from build123d import *

# Parameters (mm, degrees)
PAD_DEPTH       = 32
POCKET_DEPTH    = 27
SKETCH021_R     = 62.5
POCKET014_DEPTH = 29


with BuildPart() as part:
    # Sketch → Pad (new body)
    with BuildSketch(Plane.XY):
        with BuildLine():
            ThreePointArc((-51.234754, 40), (0, -65), (51.234754, 40))
            ThreePointArc((51.234754, 120), (37.469508, 80), (51.234754, 40))
            ThreePointArc((51.234754, 120), (0, 225), (-51.234754, 120))
            ThreePointArc((-51.234754, 40), (-37.469508, 80), (-51.234754, 120))
        make_face()
    extrude(amount=PAD_DEPTH)

    # Sketch001 (on Face6 of Pad) → Pocket (cut)
    with BuildSketch(Plane.XY.offset(32)):
        with BuildLine():
            ThreePointArc((-47.293673, 36.923008), (4.4e-05, -60), (47.293619, 36.923077))
            ThreePointArc((47.293619, 123.076923), (32.469508, 80), (47.293619, 36.923077))
            ThreePointArc((47.293619, 123.076923), (0, 220), (-47.293619, 123.076923))
            ThreePointArc((-47.293673, 36.923008), (-32.469508, 79.999956), (-47.293619, 123.076923))
        make_face()
    extrude(amount=-POCKET_DEPTH, mode=Mode.SUBTRACT)

    # Sketch021 (on Face5 of Pocket) → Pocket014 (cut)
    with BuildSketch(Plane.XY.offset(32)):
        Circle(SKETCH021_R)
    extrude(amount=-POCKET014_DEPTH, mode=Mode.SUBTRACT)


solid = part.part
Read the model definition and answer for the solid it produces. Units are mm, in the model's axes. A direction names the side the tool comes from. Round coordinates to 2 decimals unless told otherwise and drop trailing zeros. Write each loop counter-clockwise with the first axis right and the second up, starting at its lowest first coordinate (ties: lowest second). Pieces come first, ordered by that corner, then holes.
1. Which of the six approach directions +Z, -Z, +X, -X, +Y, -Y give full straight-line access (tool end or side, diameter ignored) to faces 3 (the face through (32.82, 86.98, 18.69)), 4 (the face through (38, 102, 32))?
2. Determine the mould class of faces 1 (the face through (-1, 1, 3)), 2 (the face through (-1, 82, 0)) for opening direction Y: pulls with the +Y half, pulls with the -Y half, needs draft (parallel to the pull), parting line crosses it, or undercut.
3. Given pin 1 Ø10 at (y, z) = (56, 25) entering from -X; pin 2 Ø5 at (x, y) = (-12.5, 70) entering from +Z; pin 3 Ø8 at (x, z) = (47, 16.5) entering from +Y, each flat-ended and moving along its own axis, determine where each tip first touches the part or whether it passes through.
4. Straight lines are drawn through the part: L1, parallel to Y at x = 0, z = 11; L2, parallel to Y at x = 45, z = 20.5; L3, parallel to X at y = 160, z = 26.75. For each, find the intervals that lie inside material, in ascending order.
5. The part is cut by section B-B, the plane y = 0. Determine the outline of the cut face in (x, z), then the cut area to 3 significant figures.
6. The part is cut by section C-C, the plane z = 28.5. Determine the outline of the cut face in (x, y).
7. The part is cut by section A-A, the plane x = 0. Determine the outline of the cut face in (y, z).
8. The part is cut by section D-D, the plane y = 160. Determine the outline of the cut face in (x, z).
Values:
1. face 3: +Z
1. face 4: +Z, +X, -X, +Y, -Y
2. face 1: undercut
2. face 2: needs draft
3. pin 1: stops at x = -44.3
3. pin 2: stops at z = 5
3. pin 3: stops at y = 208.74
4. L1: y = -65 to -62.5, 220 to 225
4. L2: y = -46.9 to -43.37, 43.37 to 49.63, 110.37 to 119.97, 199.69 to 206.9
4. L3: x = -65 to -60, 60 to 65
5. outline: (-65, 0) - (65, 0) - (65, 32) - (62.5, 32) - (62.5, 3) - (-62.5, 3) - (-62.5, 32) - (-65, 32) - close
5. area: 535 mm2
6. outline: (-51.23, 40) arc R65 ccw (long way) to (51.23, 40) arc R65 cw to (51.23, 120) arc R65 ccw (long way) to (-51.23, 120) arc R65 cw to start; hole (-47.29, 123.08) arc R70 cw to (-40.35, 47.73) arc R62.5 ccw (long way) to (40.35, 47.73) arc R70 cw to (47.29, 123.08) arc R60 ccw (long way) to start
7. outline: (-65, 0) - (225, 0) - (225, 32) - (220, 32) - (220, 5) - (62.5, 5) - (62.5, 3) - (-62.5, 3) - (-62.5, 32) - (-65, 32) - close
8. outline: (-65, 0) - (65, 0) - (65, 32) - (60, 32) - (60, 5) - (-60, 5) - (-60, 32) - (-65, 32) - close
